Autodesk Inventor part; units mm, degrees
ref_plane "YZ Plane" through (0, 0, 0) normal (1, 0, 0) x (0, 1, 0)
ref_plane "XZ Plane" through (0, 0, 0) normal (0, 1, 0) x (-1, 0, 0)
ref_plane "XY Plane" through (0, 0, 0) normal (0, 0, 1) x (1, 0, 0)
sketch "Sketch1" plane through (0, 0, 0) normal (0, 0, 1) x (1, 0, 0)
  arc A0 (0, 0) -> (177.8, 88.9) centre (0, 222.25) ccw
  line L0 (0, 0) -> (177.8, 0) construction
  arc A1 (0, 3.175) -> (177.8, 94.2617) centre (0, 222.25) ccw
  line L1 (0, 3.175) -> (0, 0)
  line L2 (177.8, 88.9) -> (177.8, 94.2617)
  dimension "d0" = 222.25
  dimension "d7" = 3.175
  dimension "d9" = 3.175
  dimension "d12" = 177.8
  dimension "d13" = 177.8
extrude "Extrusion1" add sketch "Sketch1" against normal blind 539.75
sketch "Sketch2" plane through (0, 0, 0) normal (0, 0, 1) x (1, 0, 0)
  arc A0 (0, 0) -> (177.8, 88.9) centre (0, 222.25) ccw
  line L0 (177.8, 88.9) -> (177.8, 232.5642)
  line L1 (177.8, 232.5642) -> (0, 222.25)
  line L2 (0, 222.25) -> (0, 0)
  dimension "d14" = 93.32
  dimension "d15" = 0
extrude "Extrusion2" add sketch "Sketch2" along normal blind 3.175
ref_plane "Work Plane1" through (0, 0, -269.875) normal (0, 0, -1) x (-1, 0, 0)
mirror "Mirror1" about plane through (0, 0, -269.875) normal (0, 0, -1) of "Extrusion2"
sketch "Sketch3" plane through (177.8, 94.2617, 0) normal (1, 0, 0) x (0, 0, -1)
  line L0 (542.925, -5.3617) -> (-3.175, -5.3617)
  line L1 (-3.175, 138.3025) -> (95.25, 138.3025)
  line L2 (95.25, 138.3025) -> (95.25, -5.3617)
  line L3 (95.25, -5.3617) -> (-3.175, -5.3617)
  line L4 (-3.175, -5.3617) -> (-3.175, 138.3025)
  line L5 (0, 138.3025) -> (-3.175, 138.3025)
  line L6 (-3.175, -5.3617) -> (-3.175, 138.3025)
  line L7 (542.925, -5.3617) -> (444.5, -5.3617)
  line L8 (444.5, -5.3617) -> (444.5, 138.3025)
  line L9 (444.5, 138.3025) -> (542.925, 138.3025)
  line L10 (542.925, 138.3025) -> (542.925, -5.3617)
  line L11 (539.75, 138.3025) -> (542.925, 138.3025)
  point P0 (0, -94.2617)
  dimension "d19" = 98.425
  dimension "d20" = 98.425
extrude "Extrusion3" add sketch "Sketch3" along normal blind 3.175
properties material "Aluminum 6061"
Design review of the part built by this model. Coordinates are the model's own, in mm. A direction names the side the tool comes from. Round coordinates to 2 decimals unless told otherwise and drop trailing zeros. Order: outer loops, then holes, each group sorted by start corner. A loop starts at its lowest first (then second) coordinate and runs counter-clockwise, first axis right, second up.
1) Consider section A-A (y = 126). State the section outline as (x, z) points (3 decimals).
The answers:
outline: (0, -542.925) - (180.975, -542.925) - (180.975, -444.5) - (177.8, -444.5) - (177.8, -539.75) - (0, -539.75) - close; (0, 0) - (177.8, 0) - (177.8, -95.25) - (180.975, -95.25) - (180.975, 3.175) - (0, 3.175) - close
2) Consider section B-B (z = -498.5). State the section outline as (x, y) points (3 decimals).
The answers:
outline: (0, 0) arc R222.25 ccw to (177.8, 88.9) - (180.975, 88.9) - (180.975, 232.564) - (177.8, 232.564) - (177.8, 94.262) arc R219.075 cw to (0, 3.175) - close
3) Machinability: for faces 1 (the flat face through (88, 119, 0)), 2 (the flat face through (92, 118, -542.925)), which of the approach directions +Z, -Z, +X, -X, +Y, -Y give a long, thin tool a straight path to every point of the face, cutting with its end or side? Answer none if there is none.
The answers:
face 1: -X, +Y
face 2: -Z, +X, -X, +Y, -Y
4) Consider section D-D (y = 76). State the section outline as (x, z) points (3 decimals), plus the area to 3 significant figures.
The answers:
outline: (0, -542.925) - (167.35, -542.925) - (167.35, 3.175) - (0, 3.175) - (0, 0) - (163.11, 0) - (163.11, -539.75) - (0, -539.75) - close
area: 3,350 mm2
5) Consider section C-C (x = 32). State the section outline as (y, z) points (3 decimals).
The answers:
outline: (2.316, -542.925) - (224.106, -542.925) - (224.106, -539.75) - (5.525, -539.75) - (5.525, 0) - (224.106, 0) - (224.106, 3.175) - (2.316, 3.175) - close
6) Clearance check with flat-ended pins moving along their axes: pin 1 Ø2 at (x, z) = (74.5, -98) entering from +Y; pin 2 Ø1 at (x, z) = (130, -200.5) entering from -Y; pin 3 Ø3.5 at (x, z) = (179, -481) entering from -Y. State where each tip first meets the part, or that it passes through.
The answers:
pin 1: stops at y = 16.6
pin 2: stops at y = 41.63
pin 3: stops at y = 88.17
7) For L1, parallel to Z at x = 111, y = 99.5 (3 decimals); L2, parallel to X at y = 101, z = -473.5 (3 decimals); L3, parallel to X at y = 55, z = -483, list the stretches that pass through material, from the lowest coordinate up.
The answers:
L1: z = -542.925 to -539.75, 0 to 3.175
L2: x = 177.8 to 180.975
L3: x = 141.5 to 146.36
